Geometry: final body of the model. Coordinates: model frame, mm. Face numbers are marked on the shaded views. A direction names the side the tool comes from. Coordinates: 2 decimals unless noted, no trailing zeros. Write each loop counter-clockwise with the first axis right and the second up, starting at its lowest first coordinate (ties: lowest second). Pieces come first, ordered by that corner, then holes. Notation, with made-up numbers: M 88,-7.5 L 136,-7.5 A16 ccw 136,23.5 Z; hole C -24.75,71 d2. An arc over 180 degrees is marked long. Write item = value, one per line. Start each with the question number.
Item 1: Section C-C on y = 1. Output: boundary loops of the cut face in (x, z).
Item 2: Section B-B on x = 55.5. Output: boundary loops of the cut face in (y, z).
Item 3: Ray query, L1, parallel to X at y = 10.25, z = 57; L2, parallel to Y at x = 54.5, z = 67. Return the intervals inside material, ascending. Write a range as [from, to].
Item 4: Section A-A on z = 60. Output: boundary loops of the cut face in (x, y).
Item 5: First-contact query: pin 1 Ø8 at (x, y) = (58, -1) entering from -Z; pin 2 Ø4 at (y, z) = (17, 43.5) entering from +X; pin 3 Ø4 at (x, z) = (51, 74) entering from +Y; pin 4 Ø4 at (x, y) = (60.5, 1.5) entering from +Z. Flat tips, straight axial feed; report the tip coordinate or a pass-through.
Item 6: Reachability of the marked faces 1 and 2 from +Z, -Z, +X, -X, +Y, -Y: full face, straight path, thin tool, end or side. Return the list, or none.
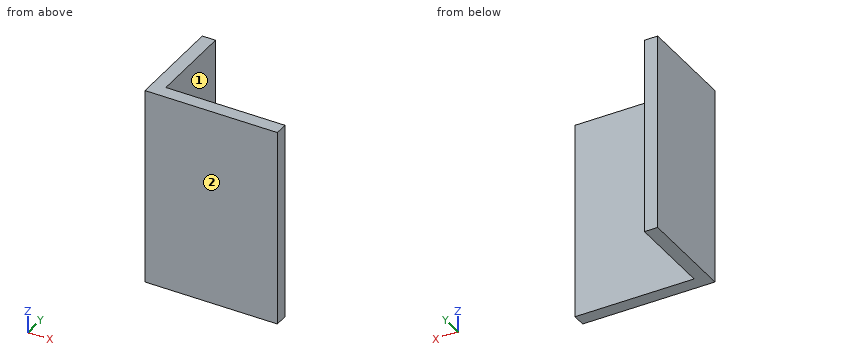
from build123d import *

# Parameters (mm, degrees)
SKETCH_1_W          = 30
SKETCH_1_H          = 15
EXTRUDE_1_DEPTH     = 20
SKETCH_2_W          = 18
SKETCH_2_H          = 13
CUT_EXTRUDE_1_DEPTH = 52.419840529
SCALE_1_SCALE       = 1.7


with BuildPart() as part:
    # 草图1 → 凸台-拉伸1 (new body)
    with BuildSketch(Plane(origin=(40, 0, 0), x_dir=(0, 0, -1), z_dir=(1, 0, 0))):
        with Locations((-35, 4.5)):
            Rectangle(SKETCH_1_W, SKETCH_1_H)
    extrude(amount=-EXTRUDE_1_DEPTH)

    # 草图2 → 切除-拉伸1 (cut, through all)
    with BuildSketch(Plane.XY.offset(50)):
        with Locations((31, 5.5)):
            Rectangle(SKETCH_2_W, SKETCH_2_H)
    extrude(amount=-CUT_EXTRUDE_1_DEPTH, mode=Mode.SUBTRACT)


with BuildPart() as part_1:
    # 缩放比例1: scaled about (0, 0, 0)
    add(part.part.scale(SCALE_1_SCALE))


solid = part_1.part
Responses:
q1.outline = M 34,34 L 37.4,34 L 37.4,85 L 34,85 Z
q2.outline = M -5.1,34 L -1.7,34 L -1.7,85 L -5.1,85 Z
q3.L1 = [34, 37.4]
q3.L2 = [-5.1, -1.7]
q4.outline = M 34,-5.1 L 68,-5.1 L 68,-1.7 L 37.4,-1.7 L 37.4,20.4 L 34,20.4 Z
q5.pin_1 = 34
q5.pin_2 = 37.4
q5.pin_3 = -1.7
q5.pin_4 = through
q6.face_1 = +Z, -Z, +X, +Y
q6.face_2 = +Z, -Z, +X, -X, -Y
